from build123d import *

# Parameters (mm, degrees)
CSK_FOR_M4_COUNTERSUNK_FLAT_HEAD_SCREW1_D           = 4.5
CSK_FOR_M4_COUNTERSUNK_FLAT_HEAD_SCREW1_CSINK_D     = 9.4
CSK_FOR_M4_COUNTERSUNK_FLAT_HEAD_SCREW1_CSINK_ANGLE = 90
CIRPATTERN1_COUNT                                   = 8


with BuildPart() as part:
    # Sketch1 → Revolve1 (revolve)
    with BuildSketch(Plane.XY, mode=Mode.PRIVATE) as revolve1_sk:
        with BuildLine():
            Line((-67, -2.5), (-67, -5))
            Line((-67, -5), (-80, -5))
            Line((-80, -5), (-80, 5))
            Line((-80, 5), (-67, 5))
            Line((-67, 5), (-67, 2.5))
            ThreePointArc((-67, 2.5), (-69.5, 0), (-67, -2.5))
        make_face()
    revolve(revolve1_sk.sketch.rotate(Axis((0, -5.61, 0), (0, 1, 0)), 270), axis=Axis((0, -5.61, 0), (0, 1, 0)))

    # CSK for M4 Countersunk Flat Head Screw1 (through all)
    with Locations(Plane(origin=(0, 5, 0), x_dir=(1, 0, 0), z_dir=(0, 1, 0))):
        with Locations((-73.5, 0)):
            csk_for_m4_countersunk_flat_head_screw1 = CounterSinkHole(CSK_FOR_M4_COUNTERSUNK_FLAT_HEAD_SCREW1_D / 2, CSK_FOR_M4_COUNTERSUNK_FLAT_HEAD_SCREW1_CSINK_D / 2, counter_sink_angle=CSK_FOR_M4_COUNTERSUNK_FLAT_HEAD_SCREW1_CSINK_ANGLE)

    # CirPattern1: CSK for M4 Countersunk Flat Head Screw1 ×8 about axis
    cirpattern1_axis = Axis((0, 0, 0), (0, 1, 0))
    for i in range(1, CIRPATTERN1_COUNT):
        add(csk_for_m4_countersunk_flat_head_screw1.rotate(cirpattern1_axis, i * 360 / CIRPATTERN1_COUNT), mode=Mode.SUBTRACT)


solid = part.part
Verification items for the finished model (mm, model axes). Give positions to 0.01 mm unless a question says otherwise; leave off trailing zeros. Order: outer loops, then holes, each group sorted by start corner. A loop starts at its lowest first (then second) coordinate and runs counter-clockwise, first axis right, second up. Notation, with made-up numbers: M 82.25,20 L 116.25,20 A19 cw 116.25,24 Z; hole C -27,79.25 d5. An arc over 180 degrees is marked long. Use one line per item in the form item = value. Start each with the question number.
Q1. Scan lines: line 1 along X through (y, z) = (-3.5, -54); line 2 along Z through (x, y) = (27, -4.5); line 3 along Z through (x, y) = (3.5, 3). Record each from-to range of solid material in increasing order. Write a range as [from, to].
Q2. Section check C-C (x = 73.5). Enter the section's corners in (y, z), then the cut area to 3 significant figures.
Q3. Go/stop test with flat-tipped pins: pin 1 Ø4 at (x, y) = (-57, 2.5) entering from +Z; pin 2 Ø4 at (x, z) = (-51.97, -51.97) entering from -Y; pin 3 Ø1 at (y, z) = (-0.5, -22) entering from -X; pin 4 Ø7 at (x, z) = (-51.97, 51.97) entering from +Y. Record where each tip stops, or that it passes through.
Q4. Section check A-A (z = 0). Enter the section's corners in (x, y).
Q5. Section check D-D (z = 73.5). Enter the section's corners in (x, y).
Q6. Mould release check, pull along Z, two halves, no side actions. Record for faces 1 (the flat face through (17, 5, -65)), 2 (the cylindrical face through (78.1, 0.07, 17.34)), 3 (the cylindrical face through (50.188, -1.278, 53.343)): +Z half, -Z half, draft (parallel to the pull), parting line (faces both ways), or undercut.
Q7. Section check B-B (x = 0). Enter the section's corners in (y, z).
Evaluation:
q1.line_1 = [-59.03, -52.95], [-51, -39.66], [39.66, 51], [52.95, 59.03]
q1.line_2 = [-75.31, -61.32], [61.32, 75.31]
q1.line_3 = [-79.92, -66.91], [66.91, 79.92]
q2.outline = M -5,-31.59 L 5,-31.59 L 5,-4.7 L 2.55,-2.25 L -5,-2.25 Z; M -5,2.25 L 2.55,2.25 L 5,4.7 L 5,31.59 L -5,31.59 Z
q2.area = 581 mm2
q3.pin_1 = 58.09
q3.pin_2 = through
q3.pin_3 = -77.06
q3.pin_4 = 3.8
q4.outline = M -80,-5 L -75.75,-5 L -75.75,2.55 L -78.2,5 L -80,5 Z; M -71.25,-5 L -67,-5 L -67,-2.5 A2.5 cw -67,2.5 L -67,5 L -68.8,5 L -71.25,2.55 Z; M 67,-5 L 71.25,-5 L 71.25,2.55 L 68.8,5 L 67,5 L 67,2.5 A2.5 cw 67,-2.5 Z; M 75.75,-5 L 80,-5 L 80,5 L 78.2,5 L 75.75,2.55 Z
q5.outline = M -31.59,-5 L -2.25,-5 L -2.25,2.55 L -4.7,5 L -31.59,5 Z; M 2.25,-5 L 31.59,-5 L 31.59,5 L 4.7,5 L 2.25,2.55 Z
q6.face_1 = draft
q6.face_2 = parting line
q6.face_3 = undercut
q7.outline = M -5,-80 L 5,-80 L 5,-78.2 L 2.55,-75.75 L -5,-75.75 Z; M -5,-71.25 L 2.55,-71.25 L 5,-68.8 L 5,-67 L 2.5,-67 A2.5 cw -2.5,-67 L -5,-67 Z; M -5,67 L -2.5,67 A2.5 cw 2.5,67 L 5,67 L 5,68.8 L 2.55,71.25 L -5,71.25 Z; M -5,75.75 L 2.55,75.75 L 5,78.2 L 5,80 L -5,80 Z
